Work out the finished part from the listing and answer in its coordinate system (mm). A direction names the side the tool comes from. Give positions to 0.01 mm unless a question says otherwise; leave off trailing zeros. Write each loop counter-clockwise with the first axis right and the second up, starting at its lowest first coordinate (ties: lowest second). Pieces come first, ordered by that corner, then holes.
1) Determine the mould class of faces 1 (the face through (2.3, -2.4, 0)), 2 (the face through (1.69, -9.64, 1.48)), 3 (the face through (1, 18.909, 2)) for opening direction Y: pulls with the +Y half, pulls with the -Y half, needs draft (parallel to the pull), parting line crosses it, or undercut.
2) A tool of negligible diameter and unlimited length cuts with its end or side. For faces 4 (the face through (2.115, -1, 2)), 5 (the face through (1, 10.909, -5)), 6 (the face through (-6.934, 18.481, 2.518)), 7 (the face through (2.713, 8.054, 3.986)), 8 (the face through (8.615, 2, 1)), from which of +Z, -Z, +X, -X, +Y, -Y can it reach the whole face along a straight path? Write none if from no direction.
3) Find section D-D (x = 6). Determine the outline of the cut face in (y, z), plus the area to 3 significant figures.
4) Find section B-B (x = 0.25). Determine the outline of the cut face in (y, z).
5) Straight lines are drawn through the part: probe 1 along Y at (x, z) = (0.5, 0.75); probe 2 along X at (y, z) = (3.5, 0.5); probe 3 along Z at (x, y) = (-6, -2). For each, find the intervals that lie inside material, in ascending order.
6) Find section A-A (y = 3). Determine the outline of the cut face in (x, z), plus the area to 3 significant figures.
7) Given pin 1 Ø2 at (x, z) = (4.5, -2.5) entering from -Y; pin 2 Ø1.8 at (x, y) = (-1, 2) entering from +Z; pin 3 Ø8 at (x, y) = (3.5, -0.5) entering from -Z, each flat-ended and moving along its own axis, determine where each tip first touches the part or whether it passes through.
Autodesk Inventor part; units mm, degrees
ref_plane "YZ Plane" through (0, 0, 0) normal (1, 0, 0) x (0, 1, 0)
ref_plane "XZ Plane" through (0, 0, 0) normal (0, 1, 0) x (-1, 0, 0)
ref_plane "XY Plane" through (0, 0, 0) normal (0, 0, 1) x (1, 0, 0)
sketch "Szkic1" plane through (0, 0, 0) normal (0, 0, 1) x (1, 0, 0)
  line L0 (-7.3846, 18.9091) -> (8.6154, 18.9091)
  line L1 (8.6154, 18.9091) -> (8.6154, -15.0909)
  line L2 (8.6154, -15.0909) -> (-7.3846, -15.0909)
  line L3 (-7.3846, -15.0909) -> (-7.3846, 18.9091)
  point P0 (0, 0)
  dimension "d1" = 16
  dimension "d2" = 34
extrude "Wyciągnięcie proste1" add sketch "Szkic1" along normal blind 5
sketch "Szkic2" plane through (0, 0, 0) normal (0, 0, -1) x (-1, 0, 0)
  line L0 (-8.6154, 18.9091) -> (7.3846, 18.9091)
  line L1 (7.3846, 18.9091) -> (7.3846, -15.0909)
  line L2 (-8.6154, 18.9091) -> (7.3846, 18.9091)
  line L3 (7.3846, 18.9091) -> (7.3846, 9.9091)
  line L4 (7.3846, 9.9091) -> (-8.6154, 9.9091)
  line L5 (-8.6154, 9.9091) -> (-8.6154, 18.9091)
  point P0 (0, 0)
  dimension "d5" = 9
extrude "Wyciągnięcie proste2" add sketch "Szkic2" along normal blind 8
chamfer "Faza1" distance 8 angle 45 1 edges at (0.6154, 18.9091, -8)
sketch "Szkic3" plane through (0, 0, 5) normal (0, 0, 1) x (1, 0, 0)
  line L0 (-2.3846, 8.9091) -> (3.6154, 8.9091)
  line L1 (3.6154, 8.9091) -> (3.6154, -12.0909)
  line L2 (3.6154, -12.0909) -> (-2.3846, -12.0909)
  line L3 (-2.3846, -12.0909) -> (-2.3846, 8.9091)
  line L4 (8.6154, 18.9091) -> (-7.3846, 18.9091)
  line L5 (-7.3846, -15.0909) -> (8.6154, -15.0909)
  line L6 (8.6154, -15.0909) -> (8.6154, 18.9091)
  point P0 (0, 0)
  dimension "d11" = 10
  dimension "d12" = 3
  dimension "d13" = 6
  dimension "d14" = 5
extrude "Wyciągnięcie proste3" cut sketch "Szkic3" against normal blind 2
sketch "Szkic4" plane through (0, 0, 3) normal (0, 0, 1) x (1, 0, 0)
  line L0 (-0.8846, 6.9091) -> (2.1154, 6.9091)
  line L1 (2.1154, 6.9091) -> (2.1154, -10.0909)
  line L2 (2.1154, -10.0909) -> (-0.8846, -10.0909)
  line L3 (-0.8846, -10.0909) -> (-0.8846, 6.9091)
  line L4 (-2.3846, 8.9091) -> (3.6154, 8.9091)
  line L5 (3.6154, 8.9091) -> (3.6154, -12.0909)
  line L6 (3.6154, -12.0909) -> (-2.3846, -12.0909)
  point P0 (0, 0)
  dimension "d17" = 2
  dimension "d19" = 3
  dimension "d20" = 1.5
  dimension "d21" = 2
extrude "Wyciągnięcie proste4" cut sketch "Szkic4" against normal up to next
fillet "Zaokrąglenie1" radius 3 4 edges at (3.6154, 8.9091, 4) (-2.3846, 8.9091, 4) (-2.3846, -12.0909, 4) (3.6154, -12.0909, 4)
fillet "Zaokrąglenie2" radius 1.5 4 edges at (-0.8846, 6.9091, 1.5) (2.1154, 6.9091, 1.5) (-0.8846, -10.0909, 1.5) (2.1154, -10.0909, 1.5)
fillet "Zaokrąglenie3" radius 1.5 4 edges at (-7.3846, -15.0909, 2.5) (8.6154, -15.0909, 2.5) (8.6154, 18.9091, 2.5) (-7.3846, 18.9091, 2.5)
sketch "Szkic5" plane through (-7.3846, 9.9091, 0) normal (0, -1, 0) x (1, 0, 0)
  line L0 (0, 0) -> (0, -8)
  line L1 (16, 0) -> (16, -8)
  line L2 (0, -8) -> (16, -8)
  line L3 (16, -8) -> (16, -4)
  line L4 (16, -4) -> (0, -4)
  line L5 (0, -4) -> (0, -8)
  line L6 (14.5, 0) -> (1.5, 0)
  point P0 (7.3846, 0)
  dimension "d28" = 4
extrude "Wyciągnięcie proste5" cut sketch "Szkic5" against normal blind 1
fillet "Zaokrąglenie5" radius 0.5 1 edges at (0.6154, 10.9091, -8)
properties part number "Trzymacz" material "Tworzywo sztuczne ABS"
Results:
1. face 1: needs draft
1. face 2: undercut
1. face 3: pulls with the +Y half
2. face 4: +Z, -Z
2. face 5: -Z, +X, -X, -Y
2. face 6: +Z, -Z, -X, +Y
2. face 7: +Z
2. face 8: +Z, -Z, +X, +Y, -Y
3. outline: (-15.09, 0) - (9.91, 0) - (9.91, -4) - (10.91, -4) - (10.91, -6.79) arc R0.5 ccw to (11.76, -7.15) - (18.91, 0) - (18.91, 5) - (-15.09, 5) - close
3. area: 206 mm2
4. outline: (-15.09, 0) - (-10.05, 0) - (-10.05, 3) - (-12.07, 3) - (-12.07, 5) - (-15.09, 5) - close; (6.86, 0) - (9.91, 0) - (9.91, -4) - (10.91, -4) - (10.91, -6.79) arc R0.5 ccw to (11.76, -7.15) - (18.91, 0) - (18.91, 5) - (8.89, 5) - (8.89, 3) - (6.86, 3) - close
5. probe 1: y = -15.09 to -10.09, 6.9 to 18.91
5. probe 2: x = -7.38 to -0.88, 2.12 to 8.62
5. probe 3: z = 0 to 5
6. outline: (-7.38, 0) - (-0.88, 0) - (-0.88, 3) - (-2.38, 3) - (-2.38, 5) - (-7.38, 5) - close; (2.12, 0) - (8.62, 0) - (8.62, 5) - (3.62, 5) - (3.62, 3) - (2.12, 3) - close
6. area: 59.0 mm2
7. pin 1: stops at y = 9.91
7. pin 2: stops at z = 3
7. pin 3: stops at z = 0
